Autodesk Inventor part; units mm, degrees
ref_plane "YZ Plane" through (0, 0, 0) normal (1, 0, 0) x (0, 1, 0)
ref_plane "XZ Plane" through (0, 0, 0) normal (0, 1, 0) x (-1, 0, 0)
ref_plane "XY Plane" through (0, 0, 0) normal (0, 0, 1) x (1, 0, 0)
sketch "Sketch1" plane through (0, 0, 0) normal (0, 0, 1) x (1, 0, 0)
  line L0 (10, 0) -> (10, 1000)
  line L1 (0, 0) -> (1181.712, 0)
  line L2 (10, 0) -> (10, 50)
  line L3 (10, 50) -> (60, 0)
  line L4 (10, 50) -> (80.7107, 50) construction
  line L5 (60, 0) -> (10, 0)
  dimension "d0" = 45
  dimension "d1" = 50
extrude "Extrusion1" add sketch "Sketch1" against normal blind 50
shell "Shell1" thickness 3 removed faces 2 at (43.3333, 16.6667, -16.6667) at (26.6667, 16.6667, -50)
sketch "Sketch2" plane through (13, 3, -3) normal (0, 1, 0) x (1, 0, 0)
  circle A0 centre (22, 22) radius 3
  line L0 (47, -3) -> (47, 47)
  line L1 (-3, 47) -> (47, -3) construction
  line L2 (-3, -3) -> (47, 47) construction
  point P0 (-13, -3)
  point P1 (22, 22)
  dimension "d5" = 6
sketch "Sketch3" plane through (13, 3, -3) normal (1, 0, 0) x (0, 0, -1)
  line L0 (-3, -3) -> (-3, 47)
  line L1 (-3, 47) -> (47.1723, -3) construction
  line L2 (47.1723, -3) -> (47.1723, 47.3451)
  line L3 (47.1723, 47.3451) -> (-3, -3) construction
  circle A0 centre (22.0861, 22.1726) radius 3
  point P0 (22.0861, 22.1726)
  dimension "d6" = 6
extrude "Extrusion2" cut sketch "Sketch2" against normal through all
extrude "Extrusion3" cut sketch "Sketch3" against normal through all
properties part number "Perfil de unión protección"
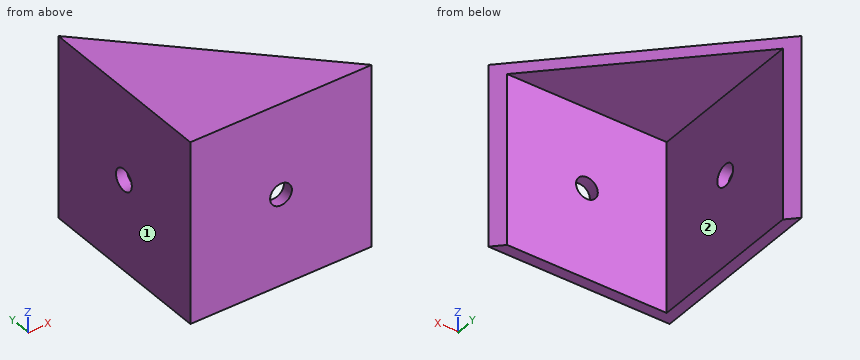
Read the model definition and answer for the solid it produces. Units are mm, in the model's axes. Face numbers are marked on the shaded views. A direction names the side the tool comes from. Round coordinates to 2 decimals unless told otherwise and drop trailing zeros. Write each loop counter-clockwise with the first axis right and the second up, starting at its lowest first coordinate (ties: lowest second). Pieces come first, ordered by that corner, then holes. Notation, with made-up numbers: (39, 41) - (82, 41) arc R23 ccw to (82, 63) - close; hole circle Ø7 at (52, 8.25). An arc over 180 degrees is marked (long way). One line per question, with ' | ' between items. Start each with the question number.
1. For the marked faces 1 and 2, determine the directions among +Z, -Z, +X, -X, +Y, -Y from which every point of the face is accessible in a straight line to the end or side of a thin tool.
2. Section D-D (z = -42) is taken. Determine the outline of the cut face in (x, y).
3. Section A-A (x = 35) is taken. Determine the outline of the cut face in (y, z).
4. Section B-B (z = -25) is taken. Determine the outline of the cut face in (x, y), and give its area (3 significant figures).
5. Section C-C (y = 33.5) is taken. Determine the outline of the cut face in (x, z), and give its area (4 significant figures).
6. Each of these flat-tipped pins is pushed along its axis until it touches: pin 1 (6 mm diameter, centred on y = 14.5, z = -45, fed in from +X); pin 2 (6 mm diameter, centred on x = 45.5, z = -7, fed in from +Y); pin 3 (13 mm diameter, centred on x = 29.5, y = 31.5, fed in from -Z). Where does it stop, or does it pass through?
7. Find the intervals of material crossed by probe 1 along Z at (x, y) = (35, 0.7); probe 2 along Z at (x, y) = (17.5, 7.5); probe 3 along X at (y, z) = (12.5, -11.5), in increasing order. Write a range as [from, to].
Filled in:
1) face 1: +Z, -Z, -X, +Y, -Y | face 2: -Z, +X, +Y
2) outline: (10, 0) - (60, 0) - (57, 3) - (13, 3) - (13, 47) - (10, 50) - close
3) outline: (0, -50) - (3, -50) - (3, -28) - (0, -28) - close; (0, -22) - (3, -22) - (3, -3) - (25, -3) - (25, 0) - (0, 0) - close
4) outline: (10, 0) - (32, 0) - (32, 3) - (13, 3) - (13, 22.17) - (10, 22.17) - close; (10, 28.17) - (13, 28.17) - (13, 47) - (10, 50) - close; (38, 0) - (60, 0) - (57, 3) - (38, 3) - close | area: 246 mm²
5) outline: (10, -50) - (13, -50) - (13, -3) - (26.5, -3) - (26.5, 0) - (10, 0) - close | area: 190.5 mm²
6) pin 1: x = 13 | pin 2: y = 3 | pin 3: z = -3
7) probe 1: [-50, -28], [-22, 0] | probe 2: [-3, 0] | probe 3: [10, 13]
